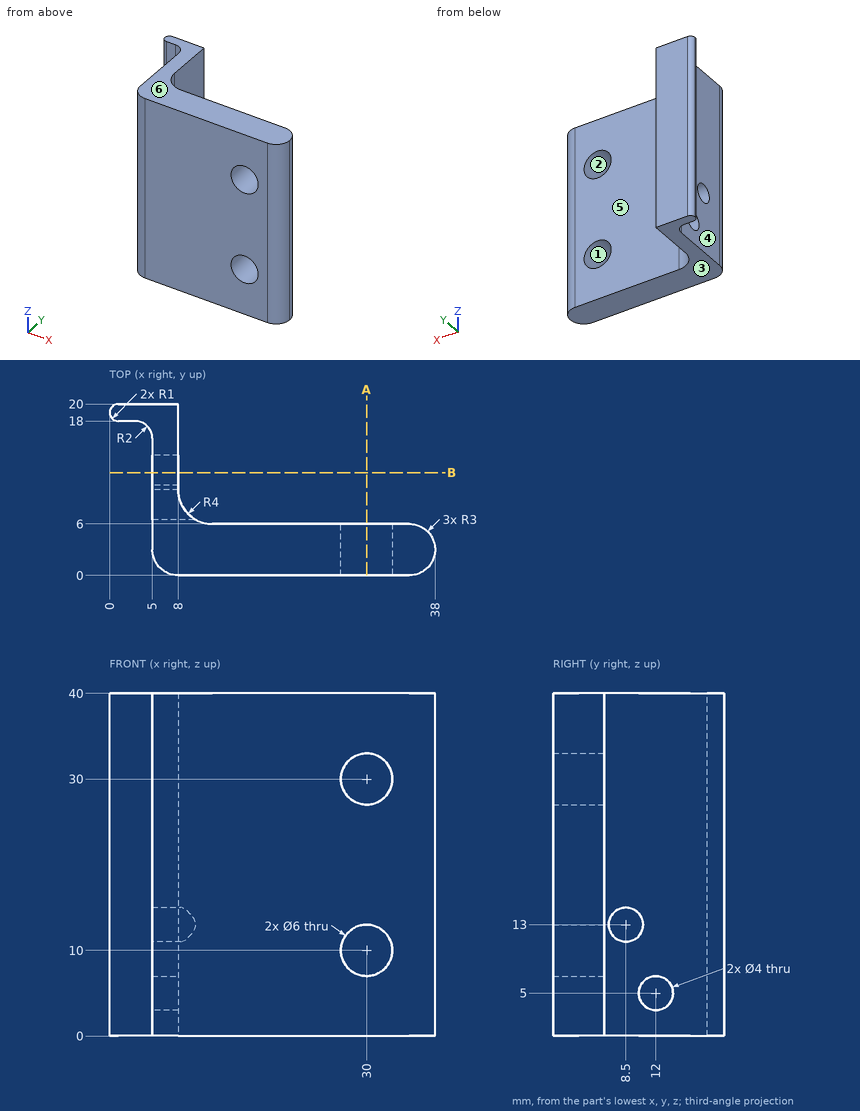
For this review, use the dimensioned drawing (mm, ordinates from the lowest corner) and the shaded views. A direction names the side the tool comes from. Coordinates: 2 decimals unless noted, no trailing zeros. Order: outer loops, then holes, each group sorted by start corner. A loop starts at its lowest first (then second) coordinate and runs counter-clockwise, first axis right, second up. Notation, with made-up numbers: M -3.75,76 L 29.25,76 A20 ccw 29.25,100 Z; hole C 12,-7.5 d2. An arc over 180 degrees is marked long. Answer as a JSON object with one key per item and string values. Group by question number.
1) Mouldability with a two-part tool opening along X and no side actions: class the marked faces 1, 2, 3 and 4 as pulls with the +X half, pulls with the -X half, needs draft (parallel to the pull), parting line crosses it, or undercut.
2) Tool access review of the marked faces 5 and 6: name each direction out of +Z, -Z, +X, -X, +Y, -Y from which nothing blocks a thin tool from reaching the whole face with its end or side.
3) Wall thickness on L1, parallel to Z at x = 30, y = 3.8; L2, parallel to Z at x = 6.7, y = 12; L3, parallel to Y at x = 14.5, z = 15: over which ranges is each line inside the solid? List them lowest first.
4) For pin 1 (8 mm diameter, centred on y = 9.5, z = 33, fed in from -X); pin 2 (5 mm diameter, centred on x = 20.5, z = 30, fed in from +Y); pin 3 (8 mm diameter, centred on y = 17, z = 4.5, fed in from +X), all flat-tipped, find the tip position at first contact; note any pin that passes through.
5) Add section B-B, the plane y = 12. Write out the cut boundary in (x, z).
6) Add section A-A, the plane x = 30. Write out the cut boundary in (y, z).
Computed values:
{
 "1": {"face 1": "undercut", "face 2": "undercut", "face 3": "needs draft", "face 4": "pulls with the -X half"},
 "2": {"face 5": "+Z, -Z, +X, +Y", "face 6": "+Z, +X, -X, +Y, -Y"},
 "3": {"L1": "z = 0 to 7, 13 to 27, 33 to 40", "L2": "z = 0 to 3, 7 to 40", "L3": "y = 0 to 6"},
 "4": {"pin 1": "stops at x = 5", "pin 2": "stops at y = 6", "pin 3": "stops at x = 8"},
 "5": {"outline": "M 5,0 L 8,0 L 8,3 L 5,3 Z; M 5,7 L 8,7 L 8,40 L 5,40 Z"},
 "6": {"outline": "M 0,0 L 6,0 L 6,7 L 0,7 Z; M 0,13 L 6,13 L 6,27 L 0,27 Z; M 0,33 L 6,33 L 6,40 L 0,40 Z"}
}
